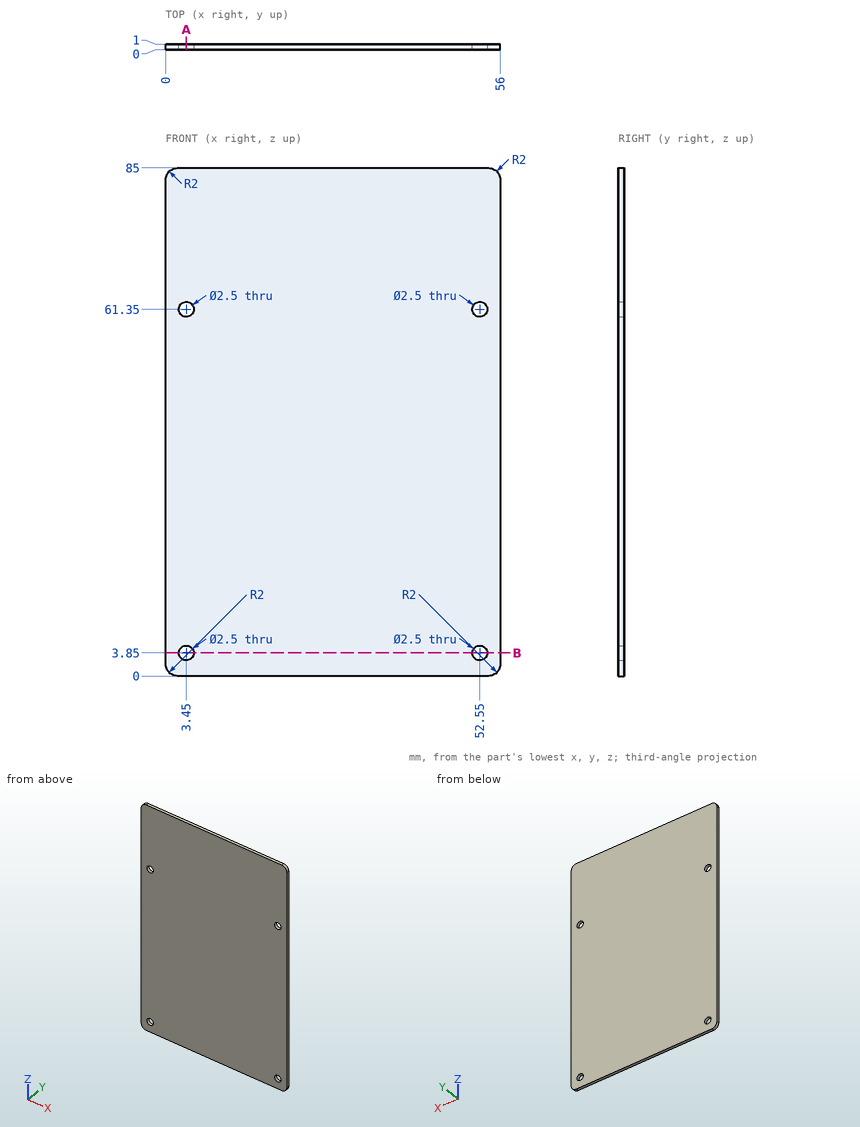
Can you work these out from the drawing? Everything is in mm from the part's minimum corner. Coordinates: 2 decimals unless noted, no trailing zeros. Loops run counter-clockwise (first coordinate to the right, second up) from the corner with the lowest first, then second, coordinate; pieces in that order, holes last. Notation, with made-up numbers: (43, 0.25) - (71, 0.25) arc R37 ccw to (71, 37.25) - close; hole circle Ø3 at (7, -34). An arc over 180 degrees is marked (long way). Put each result on its own line as item: value. Start each with the question number.
Item 1: Suppose I cut it at B-B (z = 3.85). Please give me the cut outline in (x, y), and give its area (3 significant figures).
Item 2: For pin 1 (1.5 mm diameter, centred on x = 26, z = 68, fed in from -Y), with a flat end and sliding along its axis, tell me the tip position at first contact or that it passes through.
Item 3: Suppose I cut it at A-A (x = 3.45). Please give me the cut outline in (y, z).
Item 4: If I drill on line 1 along Z through (x, y) = (52.55, 0.2); line 2 along X through (y, z) = (0.5, 61.35); line 3 along X through (y, z) = (0.95, 61), over which ranges is the centre line in solid material (lowest first)?
Here are the results:
1. outline: (0, 0) - (2.2, 0) - (2.2, 1) - (0, 1) - close; (4.7, 0) - (51.3, 0) - (51.3, 1) - (4.7, 1) - close; (53.8, 0) - (56, 0) - (56, 1) - (53.8, 1) - close
1. area: 51.0 mm²
2. pin 1: y = 0
3. outline: (0, 0) - (1, 0) - (1, 2.6) - (0, 2.6) - close; (0, 5.1) - (1, 5.1) - (1, 60.1) - (0, 60.1) - close; (0, 62.6) - (1, 62.6) - (1, 85) - (0, 85) - close
4. line 1: 0 to 2.6, 5.1 to 60.1, 62.6 to 85
4. line 2: 0 to 2.2, 4.7 to 51.3, 53.8 to 56
4. line 3: 0 to 2.25, 4.65 to 51.35, 53.75 to 56
